Autodesk Inventor part; units mm, degrees
ref_plane "Work Plane1" through (0, 10, 0) normal (0, 1, 0) x (1, 0, 0)
ref_plane "YZ Plane" through (0, 0, 0) normal (1, 0, 0) x (0, 1, 0)
ref_plane "XZ Plane" through (0, 0, 0) normal (0, 1, 0) x (-1, 0, 0)
sketch "Sketch1" plane through (0, 0, 0) normal (0, 1, 0) x (-1, 0, 0)
  circle A0 centre (0, 0) radius 12
  dimension "d0" = 24
extrude "Extrusion1" add sketch "Sketch1" along normal blind 15
ref_plane "Work Plane1" through (0, 10, 0) normal (0, 1, 0) x (1, 0, 0)
sketch "Sketch3" plane through (0, 10, 0) normal (0, 1, 0) x (1, 0, 0)
  circle A0 centre (0, 0) radius 14.5
  dimension "d5" = 29
extrude "Extrusion2" add sketch "Sketch3" against normal blind 5.75
sketch "Sketch4" plane through (0, 0, 0) normal (0, -1, 0) x (1, 0, 0)
  circle A0 centre (0, 0) radius 4.5
  dimension "d8" = 9
extrude "Extrusion3" cut sketch "Sketch4" against normal up to next
properties part number "RollerWheel"
Geometry check sheet. Reference: the model listing, model coordinates, mm. A direction names the side the tool comes from. Round coordinates to 2 decimals unless told otherwise and drop trailing zeros. Loops run counter-clockwise (first coordinate to the right, second up) from the corner with the lowest first, then second, coordinate; pieces in that order, holes last.
Item 1: Mould release check, pull along X, two halves, no side actions. Record for faces 1 (the cylindrical face through (-0.59, 7.4, 4.46)), 2 (the cylindrical face through (6.691, 7.165, 12.864)), 3 (the flat face through (2, 4.25, -12)): pulls with the +X half, pulls with the -X half, needs draft (parallel to the pull), parting line crosses it, or undercut.
Item 2: Access from +Z, -Z, +X, -X, +Y, -Y to the whole of each face (thin tool, end or side, straight path). Record for faces 4 (the cylindrical face through (11.99, 2.1, -0.53)), 5 (the flat face through (2, 10, -12)), 6 (the flat face through (-5, 0, 0)).
Item 3: Cross-section at A-A on x = 0. Record the boundary of the cut face in (y, z).
Item 4: Cross-section at B-B on z = 0. Record the boundary of the cut face in (x, y).
Item 5: Cross-section at C-C on y = 8. Record the boundary of the cut face in (x, z).
Item 6: Thickness scan on line 1 (Z direction, x = 0, y = 4.5); line 2 (Z direction, x = 0, y = 11.5); line 3 (X direction, y = 13.5, z = -1.25). Record the ranges inside material, lowest first.
Item 7: Gauge pin test, flat ends, axial feed: pin 1 (10 mm diameter, centred on x = -11.5, z = -8.5, fed in from -Y); pin 2 (4 mm diameter, centred on y = 10.5, z = 8.5, fed in from -X); pin 3 (3 mm diameter, centred on x = -6, y = 4, fed in from -Z). Record the tip position at first contact, or that the pin passes through.
Item 8: Cross-section at D-D on x = 5. Record the boundary of the cut face in (y, z), then the cut area to 3 significant figures.
Answer sheet:
1. face 1: undercut
1. face 2: parting line crosses it
1. face 3: needs draft
2. face 4: -Y
2. face 5: +Y
2. face 6: +Z, -Z, +X, -X, -Y
3. outline: (0, -12) - (4.25, -12) - (4.25, -14.5) - (10, -14.5) - (10, -12) - (15, -12) - (15, -4.5) - (0, -4.5) - close; (0, 4.5) - (15, 4.5) - (15, 12) - (10, 12) - (10, 14.5) - (4.25, 14.5) - (4.25, 12) - (0, 12) - close
4. outline: (-14.5, 4.25) - (-12, 4.25) - (-12, 0) - (-4.5, 0) - (-4.5, 15) - (-12, 15) - (-12, 10) - (-14.5, 10) - close; (4.5, 0) - (12, 0) - (12, 4.25) - (14.5, 4.25) - (14.5, 10) - (12, 10) - (12, 15) - (4.5, 15) - close
5. outline: circle Ø29 at (0, 0); hole circle Ø9 at (0, 0)
6. line 1: z = -14.5 to -4.5, 4.5 to 14.5
6. line 2: z = -12 to -4.5, 4.5 to 12
6. line 3: x = -11.93 to -4.32, 4.32 to 11.93
7. pin 1: stops at y = 0
7. pin 2: stops at x = -12.93
7. pin 3: stops at z = -13.78
8. outline: (0, -10.91) - (4.25, -10.91) - (4.25, -13.61) - (10, -13.61) - (10, -10.91) - (15, -10.91) - (15, 10.91) - (10, 10.91) - (10, 13.61) - (4.25, 13.61) - (4.25, 10.91) - (0, 10.91) - close
8. area: 358 mm2
